Check sheet for the drawn part. Datum: minimum x, y, z corner. Units: mm. A direction names the side the tool comes from. Give positions to 0.01 mm unless a question says otherwise; leave off trailing zeros. Loops run counter-clockwise (first coordinate to the right, second up) from the corner with the lowest first, then second, coordinate; pieces in that order, holes last. Notation, with made-up numbers: (-2, 79.25) - (53, 79.25) arc R29 ccw to (53, 107.25) - close; hole circle Ø10 at (0.25, 65.5). An arc over 180 degrees is marked (long way). Use one line per item in the form item = value.
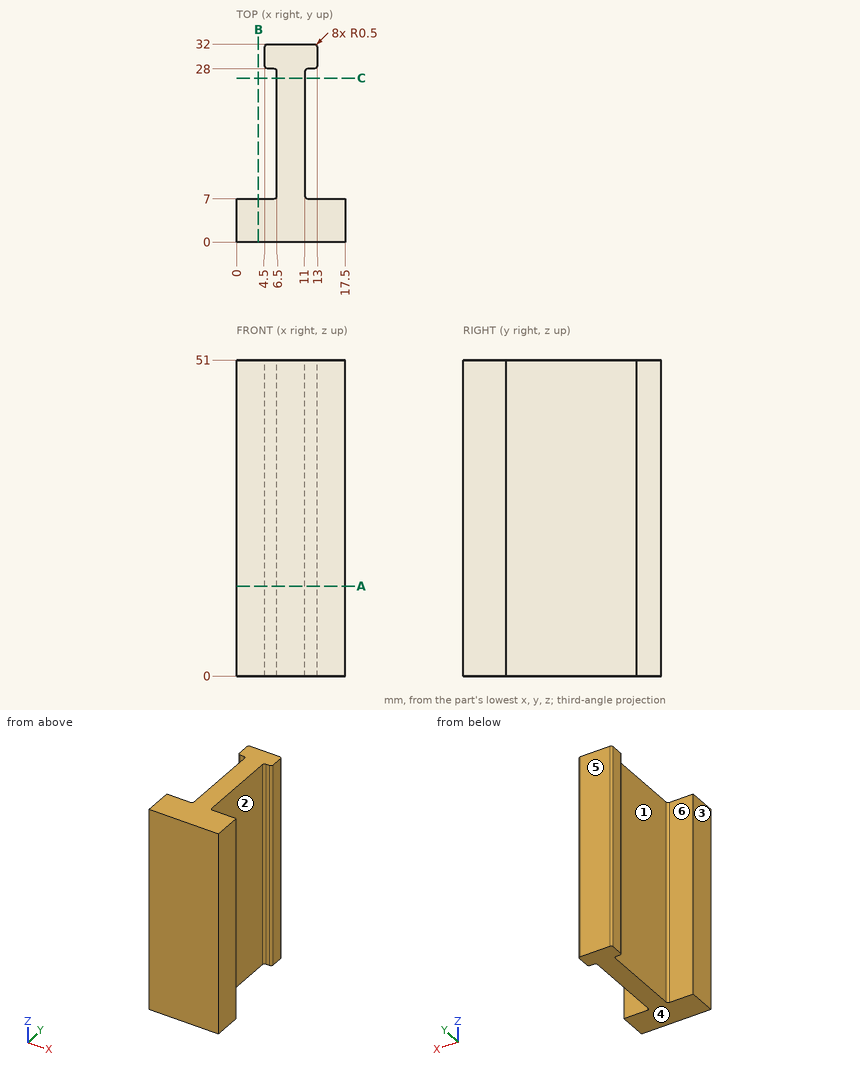
1. Section check C-C, the plane y = 26.5. Record the cut outline in (x, z), then the cut area to 4 significant figures.
Result set:
outline = (6.5, 0) - (11, 0) - (11, 51) - (6.5, 51) - close
area = 229.5 mm²
2. Scan lines: probe 1 along Y at (x, z) = (12, 46.5); probe 2 along Y at (x, z) = (16.5, 4); probe 3 along X at (y, z) = (29, 35.5). Record each from-to range of solid material in increasing order.
Result set:
probe_1 = 0 to 7, 28 to 32
probe_2 = 0 to 7
probe_3 = 4.5 to 13
3. Section check B-B, the plane x = 3.5. Record the cut outline in (y, z).
Result set:
outline = (0, 0) - (7, 0) - (7, 51) - (0, 51) - close
4. Tool access check on the marked faces 1, 2 and 3. Record the directions out of +Z, -Z, +X, -X, +Y, -Y that give a thin tool (end or side, any length) a straight path to the whole face; none if there is none.
Result set:
face_1 = +Z, -Z, -X
face_2 = +Z, -Z, +X
face_3 = +Z, -Z, -X, +Y, -Y
5. Section check A-A, the plane z = 14.5. Record the cut outline in (x, y), then the cut area to 3 significant figures.
Result set:
outline = (0, 0) - (17.5, 0) - (17.5, 7) - (11.5, 7) arc R0.5 cw to (11, 7.5) - (11, 27.5) arc R0.5 cw to (11.5, 28) - (12.5, 28) arc R0.5 ccw to (13, 28.5) - (13, 31.5) arc R0.5 ccw to (12.5, 32) - (5, 32) arc R0.5 ccw to (4.5, 31.5) - (4.5, 28.5) arc R0.5 ccw to (5, 28) - (6, 28) arc R0.5 cw to (6.5, 27.5) - (6.5, 7.5) arc R0.5 cw to (6, 7) - (0, 7) - close
area = 251 mm²
6. Depth check by flat-ended pin: pin 1 Ø1.8 at (x, z) = (15, 21) entering from +Y; pin 2 Ø10 at (y, z) = (17, 35) entering from -X; pin 3 Ø8 at (y, z) = (25.5, 42.5) entering from -X. Enter the tip coordinate at first touch or a pass-through.
Result set:
pin_1 = 7
pin_2 = 6.5
pin_3 = 4.5
7. Draft check along Y on the marked faces 4, 5 and 6. Enter one of: released by +Y, released by -Y, zero draft, split by the parting line, or undercut.
Result set:
face_4 = zero draft
face_5 = released by +Y
face_6 = undercut
